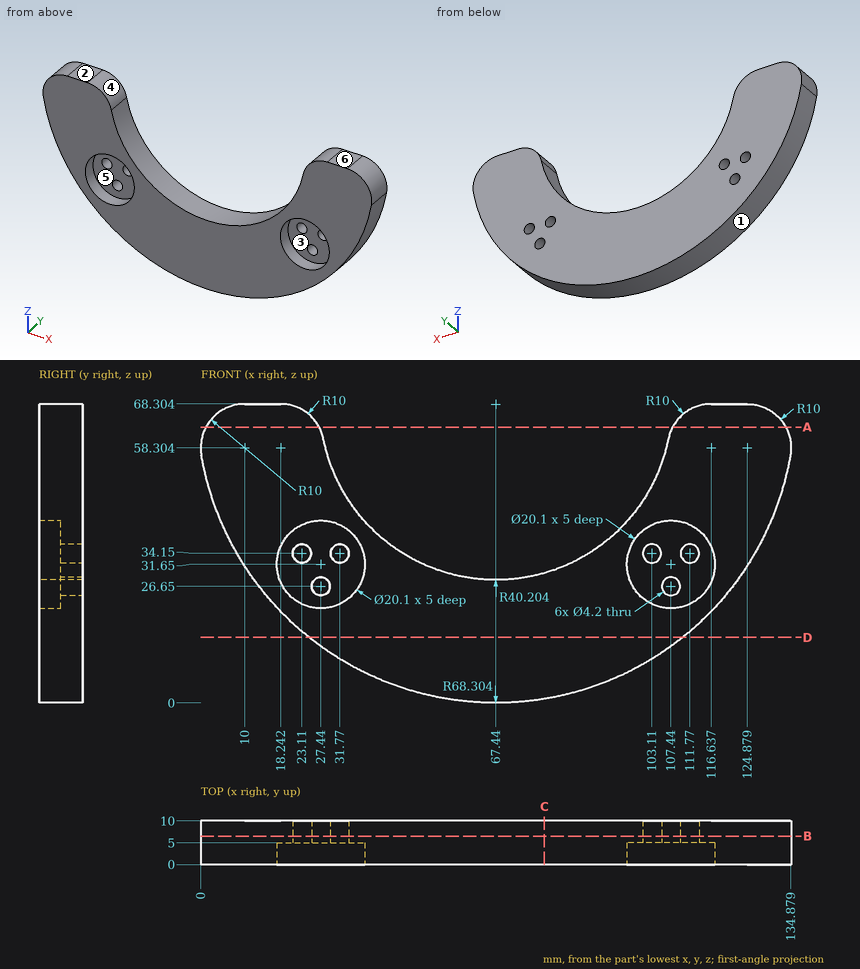
Geometry: see drawing. Coordinates: mm, zero at the bounding-box minimum. A direction names the side the tool comes from. Give positions to 0.01 mm unless a question says otherwise; leave off trailing zeros. Loops run counter-clockwise (first coordinate to the right, second up) from the corner with the lowest first, then second, coordinate; pieces in that order, holes last. Notation, with made-up numbers: (9, -32.5) - (15, -32.5) arc R26 ccw to (15, 5.5) - close; hole circle Ø7 at (40, 60.5). An arc over 180 degrees is marked (long way). Answer as CSV lines item,"result". Start each with the question number.
1. Section B-B, the plane y = 6.5. Give the number of separate pieces and of enclosed holes in the cut face, plus the area to 3 significant figures.
2. Draft query along X for the marked faces 1, 2 and 3. Return one class per face: released by +X, released by -X, zero draft, split by the parting line, or undercut.
3. Reachability of the marked faces 4, 5 and 6 from +Z, -Z, +X, -X, +Y, -Y: full face, straight path, thin tool, end or side. Return the list, or none.
4. Ray query, L1, parallel to X at y = 8.5, z = 26 (1 decimal); L2, parallel to X at y = 3.25, z = 23 (1 decimal); L3, parallel to X at y = 4, z = 57.5 (1 decimal). Return the intervals inside material, ascending.
5. Section D-D, the plane z = 15. Return loops of the section in (x, y), plus the area to 3 significant figures.
6. Pin query (flat end, axial travel): P1, Ø6, axis at y = 4, z = 8.5, coming from the +X side; P2, Ø3, axis at x = 25.5, y = 5.5, coming from the -Z side; P3, Ø5, axis at x = 111.77, z = 34.15, coming from the -Y side; P4, Ø2.5, axis at x = 27.44, z = 26.65, coming from the -Y side. Return the tip coordinate at first contact, or that it passes through.
7. Section C-C, the plane x = 78.5. Return loops of the section in (y, z).
8. Section A-A, the plane z = 63. Return loops of the section in (x, y), plus the area to 3 significant figures.
Answers:
1,separate pieces,"1"
1,enclosed holes,"6"
1,area,"4,620 mm2"
2,face 1,"split by the parting line"
2,face 2,"zero draft"
2,face 3,"undercut"
3,face 4,"+Z, +Y, -Y"
3,face 5,"-Y"
3,face 6,"+Z, +X, -X, +Y, -Y"
4,L1,"x = 13.8 to 25.4, 29.4 to 105.4, 109.4 to 121.1"
4,L2,"x = 16.3 to 22.3, 32.6 to 102.3, 112.6 to 118.6"
4,L3,"x = 0 to 28.7, 106.2 to 134.8"
5,outline,"(24.73, 0) - (110.15, 0) - (110.15, 10) - (24.73, 10) - close"
5,area,"854 mm2"
6,P1,"stops at x = 105.37"
6,P2,"stops at z = 13.26"
6,P3,"stops at y = 5"
6,P4,"passes through"
7,outline,"(0, 0.9) - (10, 0.9) - (10, 29.65) - (0, 29.65) - close"
8,outline,"(1.17, 0) - (27.07, 0) - (27.07, 10) - (1.17, 10) - close; (107.81, 0) - (133.71, 0) - (133.71, 10) - (107.81, 10) - close"
8,area,"518 mm2"
